from build123d import *

# Parameters (mm, degrees)
SKETCH1_R           = 3.9
SKETCH1_R_2         = 1.575
BOSS_EXTRUDE1_DEPTH = 30
CUT_EXTRUDE1_DEPTH  = 25
CHAMFER1_SIZE       = 0.4
CHAMFER2_SIZE       = 0.15


with BuildPart() as part:
    # Sketch1 → Boss-Extrude1 (new body)
    with BuildSketch(Plane(origin=(0, 0, 0), x_dir=(0, 0, -1), z_dir=(1, 0, 0))):
        Circle(SKETCH1_R)
        Circle(SKETCH1_R_2, mode=Mode.SUBTRACT)
    extrude(amount=BOSS_EXTRUDE1_DEPTH)

    # Sketch2 → Cut-Extrude1 (cut)
    with BuildSketch(Plane(origin=(30, 0, 0), x_dir=(0, 0, -1), z_dir=(1, 0, 0))):
        Polygon((0.506657863, 3.426849546), (-2.71440983, 2.152203353), (-3.221067693, -1.274646193), (-0.506657863, -3.426849546), (2.71440983, -2.152203353), (3.221067693, 1.274646193), align=None)
    extrude(amount=-CUT_EXTRUDE1_DEPTH, mode=Mode.SUBTRACT)

    # Chamfer1
    chamfer1_edges = [part.edges().sort_by_distance(p)[0] for p in [
        (0, 0, 3.9),
        (0, 0, 1.575),
    ]]
    chamfer(chamfer1_edges, length=CHAMFER1_SIZE)

    # Chamfer2
    chamfer2_edges = [part.edges().sort_by_distance(p)[0] for p in [
        (30, 2.350747869, -1.863862778),
        (30, 2.78952645, 1.103875984),
        (30, 0.43877858, 2.967738762),
        (30, -2.350747869, 1.863862778),
        (30, -2.78952645, -1.103875984),
        (30, -0.43877858, -2.967738762),
        (30, 0, 3.9),
    ]]
    chamfer(chamfer2_edges, length=CHAMFER2_SIZE)


solid = part.part
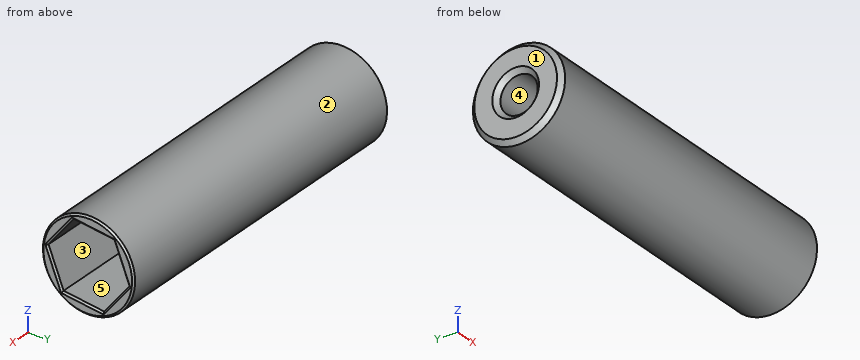
CAD build for the part. Positions are in the model's coordinates, mm. Face numbers are marked on the shaded views. A direction names the side the tool comes from. Give positions to 0.01 mm unless a question says otherwise; leave off trailing zeros. Write each loop counter-clockwise with the first axis right and the second up, starting at its lowest first coordinate (ties: lowest second). Pieces come first, ordered by that corner, then holes. Notation, with made-up numbers: M 18.5,85 L 22.5,85 A20 ccw 22.5,103 Z; hole C 48.5,86.25 d8. An arc over 180 degrees is marked long. Put each result on its own line as item: value. Start each with the question number.
(1) Probe L1, parallel to Y at x = 3.8, z = 0 (3 decimals); L2, parallel to Z at x = 21.25, y = 1.75; L3, parallel to Z at x = 7, y = 1.25. List the from-to ranges inside material, lowest first.
(2) Which spindle directions (+Z, -Z, +X, -X, +Y, -Y) get a long thin tool onto all of the face, cutting with end or side? Do the marked faces 4 and 5. Say none if no direction does.
(3) Mould opens along Y. For the marked faces 1, 2 and 3 say: +Y half, -Y half, draft (parallel to the pull), parting line (faces both ways), or undercut.
(4) Band-saw the part on B-B, the plane z = 0. Write the cut outline in (x, y) (3 decimals), and give its area (3 significant figures).
(5) Flat gauge pin, fed straight in: pin 1 Ø4 at (x, y) = (23, 2) entering from -Z. Where does the tip first touch, or does it go through?
(6) Band-saw the part on C-C, the plane y = 0. Write the cut outline in (x, z) (3 decimals).
(7) Band-saw the part on A-A, the plane x = 22.25. Write the cut outline in (y, z), and give its area (3 significant figures).
Response values:
1. L1: y = -3.9 to -1.575, 1.575 to 3.9
1. L2: z = -3.49 to -2.62, 2.77 to 3.49
1. L3: z = -3.69 to -3.22, 2.85 to 3.69
2. face 4: +X, -X
2. face 5: +X
3. face 1: draft
3. face 2: parting line
3. face 3: undercut
4. outline: M 0,-3.5 L 0.4,-3.9 L 29.85,-3.9 L 30,-3.75 L 30,-3.388 L 29.85,-3.226 L 5,-3.226 L 5,-1.575 L 0.4,-1.575 L 0,-1.975 Z; M 0,1.975 L 0.4,1.575 L 5,1.575 L 5,3.226 L 29.85,3.226 L 30,3.388 L 30,3.75 L 29.85,3.9 L 0.4,3.9 L 0,3.5 Z
4. area: 56.6 mm2
5. pin 1: stops at z = -3.9
6. outline: M 0,-3.5 L 0.4,-3.9 L 29.85,-3.9 L 30,-3.75 L 30,-3.184 L 29.85,-3.033 L 5,-3.033 L 5,-1.575 L 0.4,-1.575 L 0,-1.975 Z; M 0,1.975 L 0.4,1.575 L 5,1.575 L 5,3.033 L 29.85,3.033 L 30,3.184 L 30,3.75 L 29.85,3.9 L 0.4,3.9 L 0,3.5 Z
7. outline: C 0,0 d7.8; hole M -3.43,0.51 L -2.15,-2.71 L 1.27,-3.22 L 3.43,-0.51 L 2.15,2.71 L -1.27,3.22 Z
7. area: 16.6 mm2
